from build123d import *

# Parameters (mm, degrees)
EXTRUDE_THIN1_DEPTH = 12
SKETCH2_R           = 2.5
CUT_EXTRUDE1_DEPTH  = 28.613402543


with BuildPart() as part:
    # Sketch1 → Extrude-Thin1 (new body)
    with BuildSketch(Plane(origin=(0, 0, 0), x_dir=(1, 0, 0), z_dir=(0, 1, 0))):
        with BuildLine():
            Line((0, 21.5), (0, 9))
            ThreePointArc((0, 9), (0.878679656, 6.878679656), (3, 6))
            Line((3, 6), (9.5, 6))
            ThreePointArc((9.5, 6), (10.560660172, 5.560660172), (11, 4.5))
            Line((11, 4.5), (11, -4.5))
            ThreePointArc((11, -4.5), (10.560660172, -5.560660172), (9.5, -6))
            Line((9.5, -6), (3, -6))
            ThreePointArc((3, -6), (0.878679656, -6.878679656), (0, -9))
            Line((0, -9), (0, -21.5))
            Line((0, -21.5), (1.5, -21.5))
            Line((1.5, -21.5), (1.5, -9))
            ThreePointArc((1.5, -9), (1.939339828, -7.939339828), (3, -7.5))
            Line((3, -7.5), (9.5, -7.5))
            ThreePointArc((9.5, -7.5), (11.621320344, -6.621320344), (12.5, -4.5))
            Line((12.5, -4.5), (12.5, 4.5))
            ThreePointArc((12.5, 4.5), (11.621320344, 6.621320344), (9.5, 7.5))
            Line((9.5, 7.5), (3, 7.5))
            ThreePointArc((3, 7.5), (1.939339828, 7.939339828), (1.5, 9))
            Line((1.5, 9), (1.5, 21.5))
            Line((1.5, 21.5), (0, 21.5))
        make_face()
    extrude(amount=EXTRUDE_THIN1_DEPTH)

    # Sketch2 → Cut-Extrude1 (cut, through all)
    with BuildSketch(Plane(origin=(0, 0, 0), x_dir=(0, 0, -1), z_dir=(1, 0, 0))):
        with Locations((-15, 6)):
            Circle(SKETCH2_R)
        with Locations((15, 6)):
            Circle(SKETCH2_R)
    extrude(amount=CUT_EXTRUDE1_DEPTH, mode=Mode.SUBTRACT)


solid = part.part
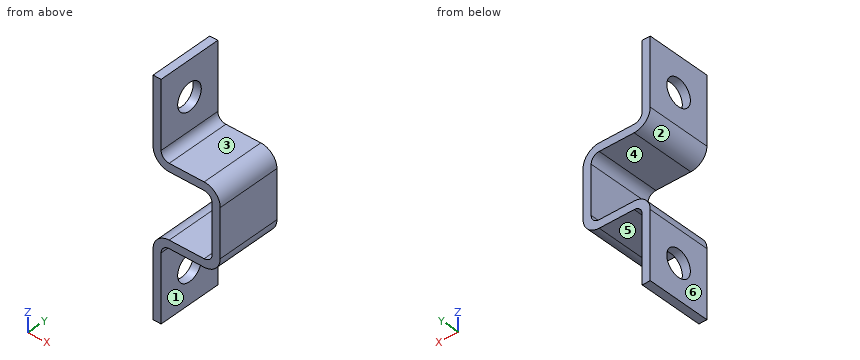
Check sheet for the modelled part. Datum: model origin and axes. Units: mm. Face numbers are marked on the shaded views. A direction names the side the tool comes from. Round coordinates to 2 decimals unless told otherwise and drop trailing zeros. Order: outer loops, then holes, each group sorted by start corner. A loop starts at its lowest first (then second) coordinate and runs counter-clockwise, first axis right, second up. Notation, with made-up numbers: M 76.5,6 L 104.5,6 A29 cw 104.5,38 Z; hole C 81.5,26 d6. An arc over 180 degrees is marked long. One line per item, written item: value. Start each with the question number.
1. Release check for a two-part mould opening along Z. For the marked faces 4, 5 and 6 record: released by +Z, released by -Z, zero draft, split by the parting line, or undercut.
2. Gauge pin test, flat ends, axial feed: P1, Ø3, axis at x = 5, y = 6.5, coming from the +Z side; P2, Ø2.5, axis at y = 8.5, z = 1, coming from the -X side; P3, Ø2, axis at x = 7, y = 4, coming from the -Z side; P4, Ø3, axis at y = 6, z = 15, coming from the -X side. Record the tip position at first contact, or that the pin passes through.
3. Scan lines: line 1 along Z through (x, y) = (0.4, 6); line 2 along Y through (x, z) = (0.4, 15); line 3 along Z through (x, y) = (0.9, 6). Record each from-to range of solid material in increasing order.
4. Section check D-D on y = 3. Enter the section's corners in (x, z).
5. Access from +Z, -Z, +X, -X, +Y, -Y to the whole of each face (thin tool, end or side, straight path). Record for the marked faces 1, 2 and 3.
6. Section check C-C on y = 6. Enter the section's corners in (x, z).
7. Section check A-A on z = -17. Enter the section's corners in (x, y), and give its area (3 significant figures).
8. Section check B-B on x = 3.5. Enter the section's corners in (y, z).
Results found:
1. face 4: undercut
1. face 5: released by -Z
1. face 6: zero draft
2. P1: z = 7.5
2. P2: x = 11
2. P3: z = -7.5
2. P4: through
3. line 1: -21.5 to -17.5, -12.5 to -7.5, 7.5 to 12.5, 17.5 to 21.5
3. line 2: 0 to 3.5, 8.5 to 12
3. line 3: -21.5 to -17.5, -12.5 to -6.86, 6.86 to 12.5, 17.5 to 21.5
4. outline: M 0,-21.5 L 1.5,-21.5 L 1.5,-9 A1.5 cw 3,-7.5 L 9.5,-7.5 A3 ccw 12.5,-4.5 L 12.5,4.5 A3 ccw 9.5,7.5 L 3,7.5 A1.5 cw 1.5,9 L 1.5,21.5 L 0,21.5 L 0,9 A3 ccw 3,6 L 9.5,6 A1.5 cw 11,4.5 L 11,-4.5 A1.5 cw 9.5,-6 L 3,-6 A3 ccw 0,-9 Z
5. face 1: -Z, +X, +Y, -Y
5. face 2: -X, +Y, -Y
5. face 3: +Z, +X, +Y, -Y
6. outline: M 0,-21.5 L 1.5,-21.5 L 1.5,-17.5 L 0,-17.5 Z; M 0,-12.5 L 1.5,-12.5 L 1.5,-9 A1.5 cw 3,-7.5 L 9.5,-7.5 A3 ccw 12.5,-4.5 L 12.5,4.5 A3 ccw 9.5,7.5 L 3,7.5 A1.5 cw 1.5,9 L 1.5,12.5 L 0,12.5 L 0,9 A3 ccw 3,6 L 9.5,6 A1.5 cw 11,4.5 L 11,-4.5 A1.5 cw 9.5,-6 L 3,-6 A3 ccw 0,-9 Z; M 0,17.5 L 1.5,17.5 L 1.5,21.5 L 0,21.5 Z
7. outline: M 0,0 L 1.5,0 L 1.5,4.5 L 0,4.5 Z; M 0,7.5 L 1.5,7.5 L 1.5,12 L 0,12 Z
7. area: 13.5 mm^2
8. outline: M 0,-7.5 L 12,-7.5 L 12,-6 L 0,-6 Z; M 0,6 L 12,6 L 12,7.5 L 0,7.5 Z
